from build123d import *

# Parameters (mm, degrees)
F1_DEPTH    = 13
F2_W        = 76.2
F2_H        = 76.2
F3_DEPTH    = 1.2
F4_R        = 1
F5_T1_DEPTH = 18.3433659759


# Not quite as in the source:
# - a fillet or chamfer that OpenCascade refuses, or shapes differently, is made with other operations: its cross-section is extruded or revolved along the edge and cut away or added


with BuildPart() as f1:
    # F0 (on Top) → F1 (new body)
    with BuildSketch(Plane.XY):
        Polygon((-36.5, 36.5), (36.5, 36.5), (38.1, 38.1), (-38.1, 38.1), (-38.1, -38.1), (38.1, -38.1), (36.5, -36.5), (-36.5, -36.5), align=None)
    extrude(amount=F1_DEPTH)

    # F2 (on Top) → F3 (join)
    with BuildSketch(Plane.XY):
        Rectangle(F2_W, F2_H)
    extrude(amount=-F3_DEPTH)

    # F4
    f4_edges = [f1.edges().sort_by_distance(p)[0] for p in [
        (0, -38.1, -1.2),
        (38.1, 0, -1.2),
        (0, 38.1, -1.2),
        (-38.1, 0, -1.2),
    ]]
    fillet(f4_edges, radius=F4_R)

    # F5: chamfer of 1 on 2 edges, made by hand

    # F5_s2 → F5_t1 (cut)
    with BuildSketch(Plane.XY.offset(-2.771682988)):
        Polygon((-37.1, -38.1), (-38.1, -37.1), (-38.1, -38.1), align=None)
        Polygon((-38.1, 37.1), (-37.1, 38.1), (-38.1, 38.1), align=None)
    extrude(amount=F5_T1_DEPTH, mode=Mode.SUBTRACT)


solid = f1.part
Build history of the part. All positions in model axes, mm. A direction names the side the tool comes from. Give positions to 0.01 mm unless a question says otherwise; leave off trailing zeros. Write each loop counter-clockwise with the first axis right and the second up, starting at its lowest first coordinate (ties: lowest second). Pieces come first, ordered by that corner, then holes. Notation, with made-up numbers: (70.5, 47.5) - (95.5, 47.5) arc R31 ccw to (95.5, 73.5) - close; hole circle Ø8 at (63, 30). An arc over 180 degrees is marked (long way). Use one line per item in the form item = value. Start each with the question number.
1. Band-saw the part on A-A on x = -33. Write the cut outline in (y, z), plus the area to 3 significant figures.
2. Band-saw the part on B-B on z = 8.75. Write the cut outline in (x, y).
3. 3-axis set-ups, long thin cutter, end or side, ignore diameter. For faces 4 (the face through (-1, 1, -1.2)), 5 (the face through (1, -36.5, 6)): which of +Z, -Z, +X, -X, +Y, -Y reach the whole face in a straight line?
4. Drop flat-ended pins along their axis: pin 1 Ø5 at (y, z) = (-15, 5.5) entering from +X; pin 2 Ø3 at (x, y) = (27, 17.5) entering from +Z. Give the stop position or say it passes through.
5. Band-saw the part on C-C on y = 11.5. Write the cut outline in (x, z), plus the area to 3 significant figures.
6. Probe line 1 (Y direction, x = -14.5, z = 4.75); line 2 (X direction, y = 32.5, z = 7); line 3 (Z direction, x = -26, y = 32). List the from-to ranges inside material, lowest first. Write a range as [from, to].
7. Two-plate mould, pull along Y, no slides. Class faces 1 (the face through (-37, 0, 13)), 2 (the face through (-36.5, -1, 6)), 3 (the face through (0, -38.1, 6)): released by +Y, released by -Y, zero draft, split by the parting line, or undercut.
Conclusion:
q1.outline = (-38.1, -0.2) arc R1 ccw to (-37.1, -1.2) - (37.1, -1.2) arc R1 ccw to (38.1, -0.2) - (38.1, 13) - (36.5, 13) - (36.5, 0) - (-36.5, 0) - (-36.5, 13) - (-38.1, 13) - close
q1.area = 133 mm²
q2.outline = (-38.1, -37.1) - (-37.1, -38.1) - (38.1, -38.1) - (36.5, -36.5) - (-36.5, -36.5) - (-36.5, 36.5) - (36.5, 36.5) - (38.1, 38.1) - (-37.1, 38.1) - (-38.1, 37.1) - close
q3.face_4 = -Z, +X, -X, +Y, -Y
q3.face_5 = +Z, +X
q4.pin_1 = -36.5
q4.pin_2 = 0
q5.outline = (-38.1, -0.2) arc R1 ccw to (-37.1, -1.2) - (37.1, -1.2) arc R1 ccw to (38.1, -0.2) - (38.1, 0) - (-36.5, 0) - (-36.5, 13) - (-38.1, 13) - close
q5.area = 112 mm²
q6.line_1 = [-38.1, -36.5], [36.5, 38.1]
q6.line_2 = [-38.1, -36.5]
q6.line_3 = [-1.2, 0]
q7.face_1 = zero draft
q7.face_2 = undercut
q7.face_3 = released by -Y
